Could you check a few things on this model? Use its own coordinates, in mm. Face numbers are marked on the shaded views. A direction names the side the tool comes from. Coordinates: 2 decimals unless noted, no trailing zeros. Order: outer loops, then holes, each group sorted by start corner. A loop starts at its lowest first (then second) coordinate and runs counter-clockwise, first axis right, second up. Notation, with made-up numbers: (79, -20) -> (119, -20) arc R36 ccw to (119, 19) -> close; hole circle Ø1 at (5, 35). An arc over 180 degrees is marked (long way). Put each result on its own line as item: value. Start each with the question number.
Q1. If we section it at C-C (z = 1.5): Please give me the cut outline in (x, y), and give its area (3 significant figures).
Q2. If we section it at D-D (x = -2.4): Please give me the cut outline in (y, z), and give its area (3 significant figures).
Q3. If we section it at A-A (x = 0): Please give me the cut outline in (y, z), and give its area (3 significant figures).
Q4. Please list where these lines run through material, in increasing order: line 1 along Y through (x, z) = (0, -3); line 2 along Y through (x, z) = (-0.35, -0.75); line 3 along X through (y, z) = (0.3, 3).
Q5. Will these pins go through, and if not, where does the flat tip stop? pin 1 (1 mm diameter, centred on x = -1, z = 2, fed in from -Y); pin 2 (2 mm diameter, centred on x = -2.5, y = 2.5, fed in from -Z).
Q6. For the marked faces 1 and 2, which set-ups out of +Z, -Z, +X, -X, +Y, -Y let a thin tool reach every point of the face, with its end or its side?
from build123d import *

# Parameters (mm, degrees)
SKETCH_2_R          = 1.85
SKETCH_2_R_2        = 1.5
EXTRUDE_1_DEPTH     = 3.15
CUT_EXTRUDE_START   = -6.3
SKETCH_3_R          = 1.5
CUT_EXTRUDE_1_DEPTH = 6.3


with BuildPart() as part:
    # 草图1 → 旋转1 (revolve)
    with BuildSketch(Plane.XY):
        with BuildLine():
            Line((0, -3), (0, 3))
            ThreePointArc((0, 3), (3, 0), (0, -3))
        make_face()
    revolve(axis=Axis((0, -3, 0), (0, 1, 0)))

    # 草图2 → 凸台-拉伸1 (add, symmetric)
    with BuildSketch(Plane.XY):
        with Locations(Location((0, 0, 0), (0, 0, 180))):
            Circle(SKETCH_2_R)
        with Locations(Location((0, 0, 0), (0, 0, 180))):
            Circle(SKETCH_2_R_2, mode=Mode.SUBTRACT)
    extrude(amount=EXTRUDE_1_DEPTH, both=True)

    # 草图3 → 切除-拉伸1 (cut)
    with BuildSketch(Plane.XY.offset(3.15).offset(CUT_EXTRUDE_START)):
        Circle(SKETCH_3_R)
    extrude(amount=CUT_EXTRUDE_1_DEPTH, mode=Mode.SUBTRACT)


solid = part.part
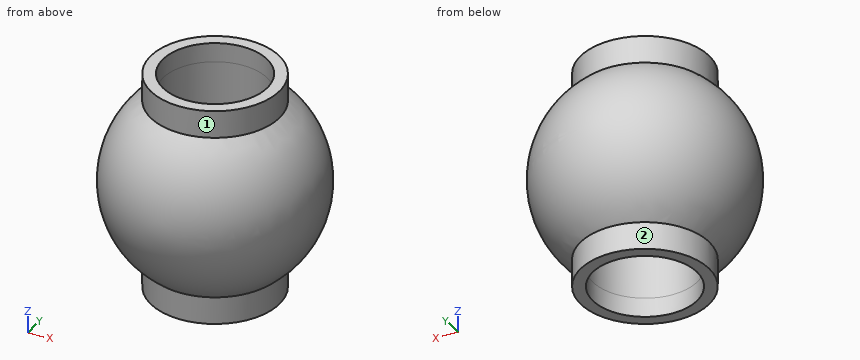
The answers:
1. outline: circle Ø5.2 at (0, 0); hole circle Ø3 at (0, 0)
1. area: 14.1 mm^2
2. outline: circle Ø3.6 at (0, 0)
2. area: 10.2 mm^2
3. outline: (-1.85, -3.15) -> (-1.5, -3.15) -> (-1.5, 3.15) -> (-1.85, 3.15) -> (-1.85, 2.36) arc R3 ccw to (-1.85, -2.36) -> close; (1.5, -3.15) -> (1.85, -3.15) -> (1.85, -2.36) arc R3 ccw to (1.85, 2.36) -> (1.85, 3.15) -> (1.5, 3.15) -> close
3. area: 12.0 mm^2
4. line 1: -1.85 to -1.5, 1.5 to 1.85
4. line 2: -2.88 to -1.46, 1.46 to 2.88
4. line 3: -1.83 to -1.47, 1.47 to 1.83
5. pin 1: y = -2.45
5. pin 2: z = -1.6
6. face 1: +Z
6. face 2: -Z
